```python
from build123d import *

# Parameters (mm, degrees)
SKIZZE1_R                                            = 23
AUFSATZ_LINEAR_AUSTRAGEN1_DEPTH                      = 5
SKIZZE2_W                                            = 4.690465157
SKIZZE2_H                                            = 4
AUFSATZ_LINEAR_AUSTRAGEN2_DEPTH                      = 5
FORMSENKUNG_F_R_M2_SENKSCHRAUBE_MIT_SCHL_D           = 2.2
FORMSENKUNG_F_R_M2_SENKSCHRAUBE_MIT_SCHL_DEPTH       = 50
FORMSENKUNG_F_R_M2_SENKSCHRAUBE_MIT_SCHL_CSINK_D     = 4.4
FORMSENKUNG_F_R_M2_SENKSCHRAUBE_MIT_SCHL_CSINK_ANGLE = 90
FORMSENKUNG_F_R_M2_SENKSCHRAUBE_MIT_SCHL_TIP         = 0.660946681


with BuildPart() as part:
    # Skizze1 → Aufsatz-Linear austragen1 (new body)
    with BuildSketch(Plane.XY):
        with BuildLine():
            Line((64.190465157, 4), (59.190465157, 4))
            ThreePointArc((59.190465157, 4), (34.007664459, 25.995043312), (7.985298356, 5))
            ThreePointArc((7.985298356, 5), (-0.004875067, 9.908732253), (-7.980769231, 4.976832421))
            ThreePointArc((-7.980769231, 4.976832421), (-33.995863589, 25.995271095), (-59.190465157, 4))
            Line((-59.190465157, 4), (-64.190465157, 4))
            Line((-64.190465157, 4), (-64.190465157, 0))
            Line((-64.190465157, 0), (-59.5, 0))
            ThreePointArc((-59.5, 0), (-33.5, -26), (-7.5, 0))
            ThreePointArc((-7.5, 0), (0, 7.5), (7.5, 0))
            ThreePointArc((7.5, 0), (33.5, -26), (59.5, 0))
            Line((59.5, 0), (64.190465157, 0))
            Line((64.190465157, 0), (64.190465157, 4))
        make_face()
        with Locations((33.5, 0)):
            Circle(SKIZZE1_R, mode=Mode.SUBTRACT)
        with Locations((-33.5, 0)):
            Circle(SKIZZE1_R, mode=Mode.SUBTRACT)
    extrude(amount=AUFSATZ_LINEAR_AUSTRAGEN1_DEPTH)

    # Skizze2 → Aufsatz-Linear austragen2 (add)
    with BuildSketch(Plane(origin=(0, 0, 0), x_dir=(-1, 0, 0), z_dir=(0, 0, -1))):
        with Locations((-61.845232579, 2)):
            Rectangle(SKIZZE2_W, SKIZZE2_H)
        with Locations((61.845232579, 2)):
            Rectangle(SKIZZE2_W, SKIZZE2_H)
    extrude(amount=AUFSATZ_LINEAR_AUSTRAGEN2_DEPTH)

    # Formsenkung für M2 Senkschraube mit Schlitz/Kreuzschlitz1
    with Locations(Plane(origin=(0, 4, 0), x_dir=(1, 0, 0), z_dir=(0, 1, 0))):
        with Locations((61.690465157, -2), (-61.690465157, -2)):
            CounterSinkHole(FORMSENKUNG_F_R_M2_SENKSCHRAUBE_MIT_SCHL_D / 2, FORMSENKUNG_F_R_M2_SENKSCHRAUBE_MIT_SCHL_CSINK_D / 2, depth=FORMSENKUNG_F_R_M2_SENKSCHRAUBE_MIT_SCHL_DEPTH, counter_sink_angle=FORMSENKUNG_F_R_M2_SENKSCHRAUBE_MIT_SCHL_CSINK_ANGLE)
            with Locations((0, 0, -(FORMSENKUNG_F_R_M2_SENKSCHRAUBE_MIT_SCHL_DEPTH + FORMSENKUNG_F_R_M2_SENKSCHRAUBE_MIT_SCHL_TIP / 2))):  # 118° drill point
                Cone(0, FORMSENKUNG_F_R_M2_SENKSCHRAUBE_MIT_SCHL_D / 2, FORMSENKUNG_F_R_M2_SENKSCHRAUBE_MIT_SCHL_TIP, mode=Mode.SUBTRACT)


solid = part.part
```
Read the model definition and answer for the solid it produces. Units are mm, in the model's axes. A direction names the side the tool comes from. Give positions to 0.01 mm unless a question says otherwise; leave off trailing zeros. Write each loop counter-clockwise with the first axis right and the second up, starting at its lowest first coordinate (ties: lowest second). Pieces come first, ordered by that corner, then holes. Notation, with made-up numbers: (-0.75, 49.5) - (27.25, 49.5) arc R19 cw to (27.25, 82.5) - close; hole circle Ø2 at (88.25, 73). An arc over 180 degrees is marked (long way). Write item = value, one per line. Start each with the question number.
Item 1: Find section C-C (y = 14.5). Give the vertices of the cut face in (x, z).
Item 2: The mould has two halves that part along Z. Classify faces 6 (the flat face through (-59.5, 2, -2)), 7 (the cylindrical face through (-62.74, 1.43, 1.67)), 8 (the flat face through (62, 2, -5)): +Z half, -Z half, draft (parallel to the pull), parting line (faces both ways), or undercut.
Item 3: Each of these flat-tipped pins is pushed along its axis until it touches: P1, Ø4, axis at x = -62.5, z = 0.5, coming from the -Y side; P2, Ø4, axis at x = 62, z = 2, coming from the +Y side; P3, Ø2, axis at x = -61.69, z = 2, coming from the +Y side; P4, Ø3, axis at y = -19.5, z = -0.5, coming from the -X side. Where does it stop, or does it pass through?
Item 4: Find section A-A (x = 33.5). Give the vertices of the cut face in (y, z), then the cut area to 3 significant figures.
Item 5: Find section D-D (x = 0). Give the vertices of the cut face in (y, z), then the cut area to 3 significant figures.
Item 6: Find section B-B (z = -3.5). Give the vertices of the cut face in (x, y).
Item 7: Find the intervals of material crossed by probe 1 along X at (y, z) = (11, 2.75); probe 2 along Y at (x, z) = (-33.5, 1.85); probe 3 along X at (y, z) = (10, 3), in increasing order. Write a range as [from, to].
Item 8: A tool of negligible diameter and unlimited length cuts with its end or side. For faces 1 (the flat face through (-62, 0, 0)), 2 (the flat face through (62, 4, -1)), 3 (the cylindrical face through (-11.562, 6.909, 2.465)), 4 (the flat face through (59.5, 2, -2)), 5 (the flat face through (62, 0, 0)), from which of +Z, -Z, +X, -X, +Y, -Y can it reach the whole face along a straight path? Write none if from no direction.
Response:
q1.outline = (-55.08, 0) - (-51.35, 0) - (-51.35, 5) - (-55.08, 5) - close; (-15.65, 0) - (-11.92, 0) - (-11.92, 5) - (-15.65, 5) - close; (11.92, 0) - (15.65, 0) - (15.65, 5) - (11.92, 5) - close; (51.35, 0) - (55.08, 0) - (55.08, 5) - (51.35, 5) - close
q2.face_6 = draft
q2.face_7 = undercut
q2.face_8 = -Z half
q3.P1 = 0
q3.P2 = 4
q3.P3 = through
q3.P4 = -52.18
q4.outline = (-26, 0) - (-23, 0) - (-23, 5) - (-26, 5) - close; (23, 0) - (26, 0) - (26, 5) - (23, 5) - close
q4.area = 30.0 mm²
q5.outline = (7.5, 0) - (9.91, 0) - (9.91, 5) - (7.5, 5) - close
q5.area = 12.0 mm²
q6.outline = (-64.19, 0) - (-59.5, 0) - (-59.5, 4) - (-64.19, 4) - close; (59.5, 0) - (64.19, 0) - (64.19, 4) - (59.5, 4) - close
q7.probe_1 = [-57.06, -53.7], [-13.3, -9.94], [9.94, 13.3], [53.7, 57.06]
q7.probe_2 = [-26, -23], [23, 26]
q7.probe_3 = [-57.5, -54.21], [-12.79, -9.5], [9.5, 12.79], [54.21, 57.5]
q8.face_1 = +Z, -Z, -X, -Y
q8.face_2 = +Z, -Z, +X, +Y
q8.face_3 = +Z, -Z
q8.face_4 = -Z, +Y, -Y
q8.face_5 = +Z, -Z, +X, -Y
